Geometry: final body of the model. Coordinates: model frame, mm. Face numbers are marked on the shaded views. Give positions to 0.01 mm unless a question says otherwise; leave off trailing zeros. Write each loop counter-clockwise with the first axis right and the second up, starting at its lowest first coordinate (ties: lowest second). Pieces come first, ordered by that corner, then holes. Notation, with made-up numbers: (76.5, 31) -> (113.5, 31) arc R12 ccw to (113.5, 40) -> close; hole circle Ø11 at (-19.75, 12.5). An arc over 180 degrees is marked (long way). Use CSV: the item, a comma, the result in double quotes. Start each with the question number.
1) Section B-B (z = -11.5). Output: boundary loops of the cut face in (x, y).
2) Contact query for flat-ended pins moving along their axis: P1, Ø1.5, axis at y = -0.5, z = 0.5, coming from the -X side; P2, Ø2, axis at x = 2, z = -8, coming from the -Y side; P3, Ø3, axis at x = -2, z = -7, coming from the +Y side. Output: stop coordinate, or through.
3) Material intervals for line 1 (Z direction, x = 0.75, y = 0); line 2 (Y direction, x = 0.75, z = -4.25); line 3 (X direction, y = -0.5, z = -4.5), sorted ascending. Write a range as [from, to].
4) Draft query along X for the marked faces 1, 2 and 3. Return one class per face: pulls with the +X half, pulls with the -X half, needs draft (parallel to the pull), parting line crosses it, or undercut.
5) Section A-A (y = 0). Output: boundary loops of the cut face in (x, z), plus the area to 3 significant figures.
```python
from build123d import *

# Parameters (mm, degrees)
SKETCH1_R           = 4
BOSS_EXTRUDE1_DEPTH = 2.3
SKETCH2_R           = 2
BOSS_EXTRUDE2_DEPTH = 13.7
CHAMFER1_SIZE       = 0.3
CUT_EXTRUDE1_DEPTH  = 2
CHAMFER2_SIZE       = 2.4


with BuildPart() as part:
    # Sketch1 → Boss-Extrude1 (new body)
    with BuildSketch(Plane.XY):
        Circle(SKETCH1_R)
    extrude(amount=BOSS_EXTRUDE1_DEPTH)

    # Sketch2 → Boss-Extrude2 (add)
    with BuildSketch(Plane(origin=(0, 0, 0), x_dir=(-1, 0, 0), z_dir=(0, 0, -1))):
        with Locations(Location((0, 0, 0), (0, 0, 180))):
            Circle(SKETCH2_R)
    extrude(amount=BOSS_EXTRUDE2_DEPTH)

    # Chamfer1
    chamfer1_edges = [part.edges().sort_by_distance(p)[0] for p in [
        (-2, 0, -13.7),
    ]]
    chamfer(chamfer1_edges, length=CHAMFER1_SIZE)

    # Sketch3 → Cut-Extrude1 (cut)
    with BuildSketch(Plane.XY.offset(2.3)):
        Polygon((0, 1.443375673), (-1.25, 0.721687836), (-1.25, -0.721687836), (0, -1.443375673), (1.25, -0.721687836), (1.25, 0.721687836), align=None)
    extrude(amount=-CUT_EXTRUDE1_DEPTH, mode=Mode.SUBTRACT)

    # Chamfer2
    # the kernel refuses this chamfer: 2.4 mm, written as the material it takes off along each edge
    with BuildSketch(Plane(origin=(0, 0, 0), x_dir=(1, 0, 0), z_dir=(0, -1, 0))) as chamfer2_piece_1_section:
        Polygon((4 - CHAMFER2_SIZE, 0), (4, CHAMFER2_SIZE), (4, 0), align=None)
    chamfer2_piece_1 = revolve(axis=Axis((0, 0, 0), (0, 0, 1)), mode=Mode.PRIVATE)
    chamfer2_piece_1 = chamfer2_piece_1 - Plane(origin=(0, 0, 1.405884102), x_dir=(1, 0, 0), z_dir=(0, 0, 1)) * Cylinder(2, 16, mode=Mode.PRIVATE)
    add(chamfer2_piece_1, mode=Mode.SUBTRACT)


solid = part.part
```
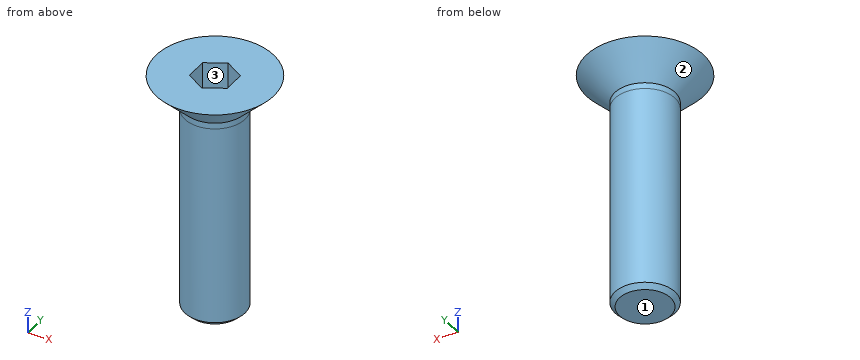
Answers follow:
1,outline,"circle Ø4 at (0, 0)"
2,P1,"stops at x = -2.82"
2,P2,"stops at y = -1.73"
2,P3,"stops at y = 1.94"
3,line 1,"z = [-13.7, 0.3]"
3,line 2,"y = [-1.85, 1.85]"
3,line 3,"x = [-1.94, 1.94]"
4,face 1,"needs draft"
4,face 2,"parting line crosses it"
4,face 3,"undercut"
5,outline,"(-3.9, 2.3) -> (-2, 0.4) -> (-2, -13.4) -> (-1.7, -13.7) -> (1.7, -13.7) -> (2, -13.4) -> (2, 0.4) -> (3.9, 2.3) -> (1.25, 2.3) -> (1.25, 0.3) -> (-1.25, 0.3) -> (-1.25, 2.3) -> close"
5,area,"62.5 mm^2"
